from build123d import *

# Parameters (mm, degrees)
F1_DEPTH = 3.175
F2_R     = 5.08
F4_D     = 6.35


with BuildPart() as f1:
    # F0 (on Front) → F1 (new body)
    with BuildSketch(Plane.XZ):
        Polygon((-38.1, 25.4), (-38.1, 0), (38.1, 0), (38.1, 25.4), (12.7, 76.2), (-12.7, 76.2), align=None)
    extrude(amount=F1_DEPTH)

    # F2
    f2_edges = [f1.edges().sort_by_distance(p)[0] for p in [
        (12.7, -1.5875, 76.2),
        (-12.7, -1.5875, 76.2),
        (38.1, -1.5875, 25.4),
        (38.1, -1.5875, 0),
        (-38.1, -1.5875, 25.4),
        (-38.1, -1.5875, 0),
    ]]
    fillet(f2_edges, radius=F2_R)

    # F4 (through all)
    with Locations(Plane(origin=(0, 0, 0), x_dir=(-1, 0, 0), z_dir=(0, 1, 0))):
        with Locations((-25.4, 12.7), (0, 12.7), (25.4, 12.7), (0, 38.1), (0, 63.5)):
            Hole(F4_D / 2)


solid = f1.part
Model file for the job. Use its own axes, mm. Give positions to 0.01 mm unless a question says otherwise; leave off trailing zeros. Order: outer loops, then holes, each group sorted by start corner. A loop starts at its lowest first (then second) coordinate and runs counter-clockwise, first axis right, second up. Notation, with made-up numbers: (5, 87) - (23, 87) arc R17 cw to (23, 95) - close; hole circle Ø4 at (-39, -35). An arc over 180 degrees is marked (long way). One line per item, written item: value.
Item 1: Slice it at C-C (z = 38.1). List the corners of the cut face in (x, y) (3 decimals).
Response values:
outline: (-31.75, -3.175) - (-3.175, -3.175) - (-3.175, 0) - (-31.75, 0) - close; (3.175, -3.175) - (31.75, -3.175) - (31.75, 0) - (3.175, 0) - close
Item 2: Slice it at D-D (x = 0). List the corners of the cut face in (y, z) (3 decimals).
Response values:
outline: (-3.175, 0) - (0, 0) - (0, 9.525) - (-3.175, 9.525) - close; (-3.175, 15.875) - (0, 15.875) - (0, 34.925) - (-3.175, 34.925) - close; (-3.175, 41.275) - (0, 41.275) - (0, 60.325) - (-3.175, 60.325) - close; (-3.175, 66.675) - (0, 66.675) - (0, 76.2) - (-3.175, 76.2) - close
Item 3: Slice it at A-A (x = -25.4). List the corners of the cut face in (y, z) (3 decimals), then the cut area to 3 significant figures.
Response values:
outline: (-3.175, 0) - (0, 0) - (0, 9.525) - (-3.175, 9.525) - close; (-3.175, 15.875) - (0, 15.875) - (0, 50.8) - (-3.175, 50.8) - close
area: 141 mm2
Item 4: Two-plate mould, pull along X, no slides. Class faces 1 (the flat face through (-1, -3.175, 30)), 2 (the cylindrical face through (1.707, -1.61, 66.177)), 3 (the flat face through (26, -1.6, 49.6)), 4 (the cylindrical face through (-12.2, -1.61, 75.46)): released by +X, released by -X, zero draft, split by the parting line, or undercut.
Response values:
face 1: zero draft
face 2: undercut
face 3: released by +X
face 4: released by -X
Item 5: Wall check: line 1 (Z direction, x = 0, y = -1.7) (3 decimals); line 2 (Z direction, x = -24, y = -2.45); line 3 (Z direction, x = -22.5, y = -2.75). Give the ranges that are in metal, low to high.
Response values:
line 1: 0 to 9.525, 15.875 to 34.925, 41.275 to 60.325, 66.675 to 76.2
line 2: 0 to 9.85, 15.55 to 53.6
line 3: 0 to 11.41, 13.99 to 56.6
Item 6: Slice it at B-B (y = -0.95). List the corners of the cut face in (x, z) (3 decimals), then the cut area to 3 significant figures.
Response values:
outline: (-38.1, 5.08) arc R5.08 ccw to (-33.02, 0) - (33.02, 0) arc R5.08 ccw to (38.1, 5.08) - (38.1, 24.201) arc R5.08 ccw to (37.564, 26.473) - (14.104, 73.392) arc R5.08 ccw to (9.56, 76.2) - (-9.56, 76.2) arc R5.08 ccw to (-14.104, 73.392) - (-37.564, 26.473) arc R5.08 ccw to (-38.1, 24.201) - close; hole circle Ø6.35 at (-25.4, 12.7); hole circle Ø6.35 at (0, 12.7); hole circle Ø6.35 at (0, 38.1); hole circle Ø6.35 at (0, 63.5); hole circle Ø6.35 at (25.4, 12.7)
area: 4,340 mm2
